from build123d import *

# Parameters (mm, degrees)
EXTRUDE_1_DEPTH     = 2
SKETCH_2_W          = 3
SKETCH_2_H          = 25
EXTRUDE_2_DEPTH     = 8
SKETCH_3_R          = 1.85
CUT_EXTRUDE_1_DEPTH = 8


with BuildPart() as part:
    # 草图1 → 凸台-拉伸1 (new body)
    with BuildSketch(Plane(origin=(0, 0, 0), x_dir=(1, 0, 0), z_dir=(0, 1, 0))):
        Polygon((26, 30), (-26, 30), (-26, 60), (-116, 60), (-136, 0), (-95, -90), (95, -90), (136, 0), (116, 60), (26, 60), align=None)
    extrude(amount=EXTRUDE_1_DEPTH)

    # 草图2 → 凸台-拉伸2 (add)
    with BuildSketch(Plane(origin=(0, 2, 0), x_dir=(1, 0, 0), z_dir=(0, 1, 0))):
        with Locations((27.5, 47.5)):
            Rectangle(SKETCH_2_W, SKETCH_2_H)
        with Locations((-27.5, 47.5)):
            Rectangle(SKETCH_2_W, SKETCH_2_H)
    extrude(amount=EXTRUDE_2_DEPTH)

    # 草图3 → 切除-拉伸1 (cut)
    with BuildSketch(Plane.ZY.offset(-26)):
        with Locations((-47.5, 6)):
            Circle(SKETCH_3_R)
    extrude(amount=-CUT_EXTRUDE_1_DEPTH, mode=Mode.SUBTRACT)


solid = part.part
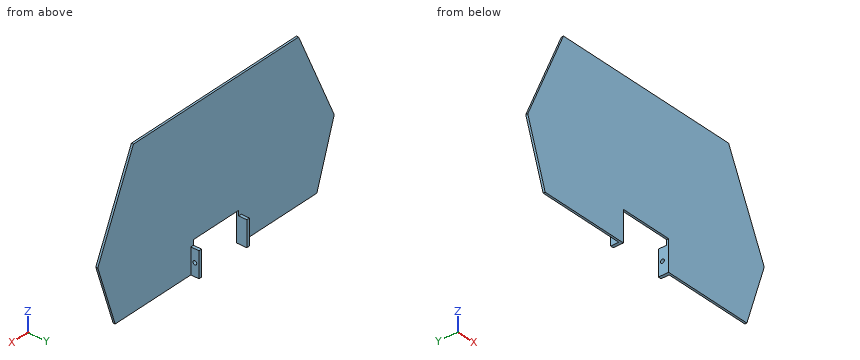
CAD build for the part. Positions are in the model's coordinates, mm. Round coordinates to 2 decimals unless told otherwise and drop trailing zeros. Write each loop counter-clockwise with the first axis right and the second up, starting at its lowest first coordinate (ties: lowest second). Pieces come first, ordered by that corner, then holes.
(1) Slice it at A-A, the plane y = 6. Write the cut outline in (x, z).
(2) Slice it at C-C, the plane z = 17.5. Write the cut outline in (x, y), and give its area (3 significant figures).
(3) Probe line 1 along X through (y, z) = (7, -51); line 2 along Y through (x, z) = (28.1, -47.5); line 3 along Y through (x, z) = (78, -14). List the from-to ranges inside material, lowest first.
(4) Drop flat-ended pins along their axis: P1, Ø5, axis at y = 5.5, z = -41.5, coming from the +X side; P2, Ø1.5, axis at x = -28, y = 6, coming from the +Z side; P3, Ø10, axis at x = -22, z = 35.5, coming from the +Y side. Give the stop position or say it passes through.
(5) Slice it at B-B, the plane x = 5. Write the cut outline in (y, z), and give its area (3 significant figures).
From the geometry:
1. outline: (-29, -60) - (-26, -60) - (-26, -35) - (-29, -35) - close; (26, -60) - (29, -60) - (29, -49.35) - (26, -49.35) - close; (26, -45.65) - (29, -45.65) - (29, -35) - (26, -35) - close
2. outline: (-128.03, 0) - (128.03, 0) - (128.03, 2) - (-128.03, 2) - close
2. area: 512 mm2
3. line 1: x = -29 to -26, 26 to 29
3. line 2: y = 0 to 4.15, 7.85 to 10
3. line 3: y = 0 to 2
4. P1: stops at x = 29
4. P2: stops at z = -35
4. P3: stops at y = 2
5. outline: (0, -30) - (2, -30) - (2, 90) - (0, 90) - close
5. area: 240 mm2
